```python
from build123d import *

# Parameters (mm, degrees)
SKETCH1_W           = 29
SKETCH1_H           = 30
BOSS_EXTRUDE1_DEPTH = 29
SKETCH2_R           = 14.5
BOSS_EXTRUDE2_DEPTH = 11.78
SKETCH3_R           = 1.2
CUT_EXTRUDE1_DEPTH  = 2.5
SKETCH4_R           = 4.5
BOSS_EXTRUDE3_DEPTH = 6
SKETCH5_R           = 28.5
BOSS_EXTRUDE4_DEPTH = 58


with BuildPart() as part:
    # Sketch1 → Boss-Extrude1 (new body)
    with BuildSketch(Plane(origin=(0, 0, 0), x_dir=(1, 0, 0), z_dir=(0, 1, 0))):
        Rectangle(SKETCH1_W, SKETCH1_H)
    extrude(amount=BOSS_EXTRUDE1_DEPTH)

    # Sketch2 → Boss-Extrude2 (add)
    with BuildSketch(Plane.XY.offset(15)):
        with Locations((0, 14.5)):
            Circle(SKETCH2_R)
    extrude(amount=BOSS_EXTRUDE2_DEPTH)

    # Sketch3 → Cut-Extrude1 (cut)
    with BuildSketch(Plane.XZ):
        with Locations((-10, 12)):
            Circle(SKETCH3_R)
        with Locations((10, 12)):
            Circle(SKETCH3_R)
        with Locations((0, -11.5)):
            Circle(SKETCH3_R)
    extrude(amount=-CUT_EXTRUDE1_DEPTH, mode=Mode.SUBTRACT)

    # Sketch4 → Boss-Extrude3 (add)
    with BuildSketch(Plane(origin=(0, 0, -15), x_dir=(-1, 0, 0), z_dir=(0, 0, -1))):
        with Locations((-8.5, 23)):
            Circle(SKETCH4_R)
    extrude(amount=BOSS_EXTRUDE3_DEPTH)

    # Sketch5 → Boss-Extrude4 (add)
    with BuildSketch(Plane.XY.offset(26.78)):
        with Locations((0, 14.5)):
            Circle(SKETCH5_R)
    extrude(amount=BOSS_EXTRUDE4_DEPTH)


solid = part.part
```
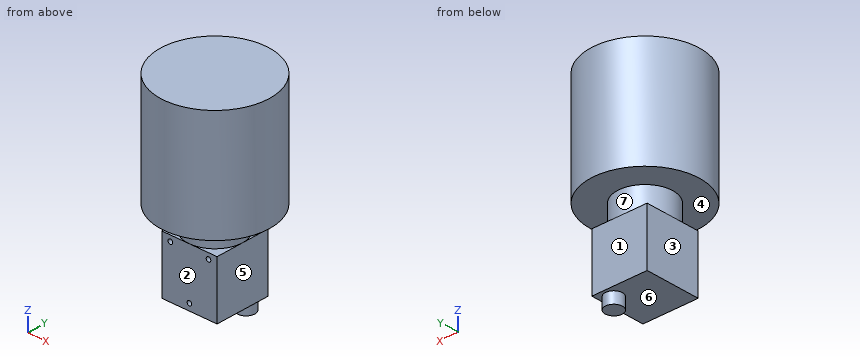
Work out the finished part from the listing and answer in its coordinate system (mm). Face numbers are marked on the shaded views. A direction names the side the tool comes from. Round coordinates to 2 decimals unless told otherwise and drop trailing zeros. Loops run counter-clockwise (first coordinate to the right, second up) from the corner with the lowest first, then second, coordinate; pieces in that order, holes last. Notation, with made-up numbers: M -34,29 L -14,29 A23 ccw -14,37 Z; hole C -27,-40 d9. An arc over 180 degrees is marked long. Use CSV: the item, a comma, the result in double quotes.
Q1. Consider L1, parallel to Z at x = -7.5, y = 1; L2, parallel to X at y = 14, z = 60; L3, parallel to X at y = 14, z = 12. Determine where each line is inside the solid, lowest interval first.
Determined:
L1,"-15 to 15, 26.78 to 84.78"
L2,"-28.5 to 28.5"
L3,"-14.5 to 14.5"
Q2. Section B-B, the plane x = 2.5 is taken. Determine the outline of the cut face in (y, z).
Determined:
outline,"M -13.89,26.78 L 0.22,26.78 L 0.22,15 L 0,15 L 0,-15 L 29,-15 L 29,15 L 28.78,15 L 28.78,26.78 L 42.89,26.78 L 42.89,84.78 L -13.89,84.78 Z"
Q3. Section C-C, the plane y = 23 is taken. Determine the outline of the cut face in (x, z), then the cut area to 3 significant figures.
Determined:
outline,"M -27.2,26.78 L -11.75,26.78 L -11.75,15 L -14.5,15 L -14.5,-15 L 4,-15 L 4,-21 L 13,-21 L 13,-15 L 14.5,-15 L 14.5,15 L 11.75,15 L 11.75,26.78 L 27.2,26.78 L 27.2,84.78 L -27.2,84.78 Z"
area,"4,360 mm2"
Q4. A tool of negligible diameter and unlimited length cuts with its end or side. For the marked faces 1, 2, 3 and 4, from which of +Z, -Z, +X, -X, +Y, -Y can it reach the whole face along a straight path? Write none if from no direction.
Determined:
face 1,"-Z, +X, -X, +Y"
face 2,"-Z, +X, -X, -Y"
face 3,"-Z, -X, +Y, -Y"
face 4,"none"
Q5. Each of these flat-tipped pins is pushed along its axis until it touches: pin 1 (3 mm diameter, centred on x = -10, z = 12, fed in from +Y); pin 2 (12 mm diameter, centred on x = -1, z = 14, fed in from -Y); pin 3 (10 mm diameter, centred on x = 15, z = 46.5, fed in from +Y). Where does it stop, or does it pass through?
Determined:
pin 1,"y = 29"
pin 2,"y = 0"
pin 3,"y = 41.19"
Q6. Section D-D, the plane x = -10 is taken. Determine the outline of the cut face in (y, z).
Determined:
outline,"M -12.19,26.78 L 4,26.78 L 4,15 L 0,15 L 0,13.2 L 2.5,13.2 L 2.5,10.8 L 0,10.8 L 0,-15 L 29,-15 L 29,15 L 25,15 L 25,26.78 L 41.19,26.78 L 41.19,84.78 L -12.19,84.78 Z"
Q7. Section A-A, the plane z = -11.5 is taken. Determine the outline of the cut face in (x, y).
Determined:
outline,"M -14.5,0 L -1.2,0 L -1.2,2.5 L 1.2,2.5 L 1.2,0 L 14.5,0 L 14.5,29 L -14.5,29 Z"
Q8. The mould has two halves that part along Z. Classify the marked faces 5, 6 and 7: pulls with the +Z half, pulls with the -Z half, needs draft (parallel to the pull), parting line crosses it, or undercut.
Determined:
face 5,"needs draft"
face 6,"pulls with the -Z half"
face 7,"undercut"
